Can you work these out from the drawing? Everything is in mm from the part's minimum corner. A direction names the side the tool comes from. Coordinates: 2 decimals unless noted, no trailing zeros. Order: outer loops, then holes, each group sorted by start corner. A loop starts at its lowest first (then second) coordinate and runs counter-clockwise, first axis right, second up. Notation, with made-up numbers: (5.25, 82.5) -> (30.25, 82.5) arc R29 cw to (30.25, 113.5) -> close; hole circle Ø2 at (48.5, -36). An arc over 180 degrees is marked (long way). Use a Markdown table: item, result. Add a question column.
1) Which directions (+Z, -Z, +X, -X, +Y, -Y) give clear straight access to the entire face, cutting with the end or side of a thin tool? Please do the marked faces 3, 4 and 5.
2) If we section it at D-D (x = 63.5): Write out the boundary of the cut face in (y, z), plus the area to 3 significant figures.
3) Thinking about a two-plate mould opening in X: for the marked faces 1 and 2, which applies, +X half, -X half, draft (parallel to the pull), parting line (faces both ways), or undercut?
4) If we section it at A-A (z = 17): Write out the boundary of the cut face in (x, y), plus the area to 3 significant figures.
5) If we section it at C-C (z = 29.5): Write out the boundary of the cut face in (x, y), plus the area to 3 significant figures.
6) If we section it at B-B (y = 2.75): Write out the boundary of the cut face in (x, z), plus the area to 3 significant figures.
7) If I drill on L1, parallel to X at y = 7, z = 26.5; L2, parallel to X at y = 2, z = 31; L3, parallel to X at y = 2.25, z = 19 (1 decimal), over which ranges is the centre line in solid material (lowest first)? Write a range as [from, to].
8) Will these pins go through, and if not, where does the flat tip stop? pin 1 Ø3 at (x, y) = (76, 2.5) entering from -Z; pin 2 Ø2.5 at (y, z) = (4.5, 28.5) entering from -X; pin 3 Ø2.5 at (y, z) = (2.5, 31.5) entering from -X; pin 4 Ø5 at (x, z) = (63, 4.5) entering from -Y.
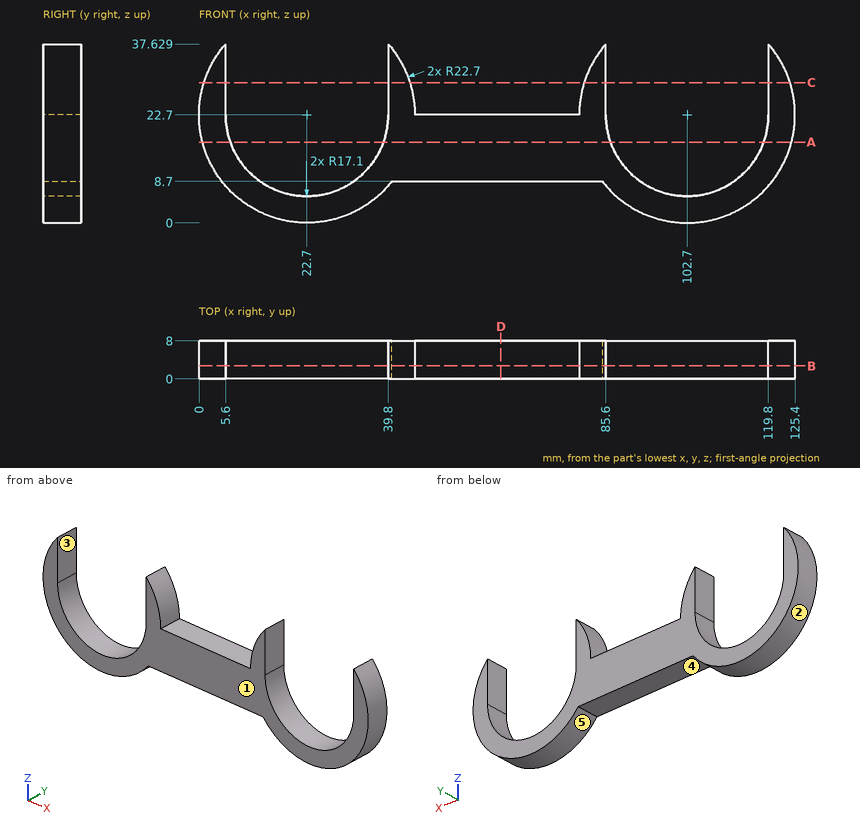
Answer sheet:
| question | item | result |
|---|---|---|
| 1 | face 3 | +Z, +Y, -Y |
| 1 | face 4 | -Z, +Y, -Y |
| 1 | face 5 | +Y, -Y |
| 2 | outline | (0, 8.7) -> (8, 8.7) -> (8, 22.7) -> (0, 22.7) -> close |
| 2 | area | 112 mm2 |
| 3 | face 1 | draft |
| 3 | face 2 | undercut |
| 4 | outline | (0.73, 0) -> (6.58, 0) -> (6.58, 8) -> (0.73, 8) -> close; (38.82, 0) -> (86.58, 0) -> (86.58, 8) -> (38.82, 8) -> close; (118.82, 0) -> (124.67, 0) -> (124.67, 8) -> (118.82, 8) -> close |
| 4 | area | 476 mm2 |
| 5 | outline | (1.04, 0) -> (5.6, 0) -> (5.6, 8) -> (1.04, 8) -> close; (39.8, 0) -> (44.36, 0) -> (44.36, 8) -> (39.8, 8) -> close; (81.04, 0) -> (85.6, 0) -> (85.6, 8) -> (81.04, 8) -> close; (119.8, 0) -> (124.36, 0) -> (124.36, 8) -> (119.8, 8) -> close |
| 5 | area | 146 mm2 |
| 6 | outline | (5.6, 22.7) -> (5.6, 37.63) arc R22.7 ccw (long way) to (40.57, 8.7) -> (84.83, 8.7) arc R22.7 ccw (long way) to (119.8, 37.63) -> (119.8, 22.7) arc R17.1 cw to (85.6, 22.7) -> (85.6, 37.63) arc R22.7 ccw to (80, 22.7) -> (45.4, 22.7) arc R22.7 ccw to (39.8, 37.63) -> (39.8, 22.7) arc R17.1 cw to start |
| 6 | area | 1,460 mm2 |
| 7 | L1 | [0.32, 5.6], [39.8, 45.08], [80.32, 85.6], [119.8, 125.08] |
| 7 | L2 | [1.57, 5.6], [39.8, 43.83], [81.57, 85.6], [119.8, 123.83] |
| 7 | L3 | [0.3, 6], [39.4, 86], [119.4, 125.1] |
| 8 | pin 1 | z = 8.7 |
| 8 | pin 2 | x = 0.46 |
| 8 | pin 3 | x = 1.29 |
| 8 | pin 4 | through |
